from build123d import *

# Parameters (mm, degrees)
BOSS_EXTRUDE1_DEPTH = 15
FILLET1_R           = 5
FILLET2_R           = 5
SKETCH4_W           = 5
SKETCH4_H           = 5
BOSS_EXTRUDE2_DEPTH = 15
SKETCH6_W           = 15
SKETCH6_H           = 35
BOSS_EXTRUDE3_DEPTH = 5
FILLET3_R           = 5
CHAMFER1_SIZE       = 10
BOSS_EXTRUDE4_DEPTH = 5
SKETCH9_R           = 8
CUT_EXTRUDE6_DEPTH  = 5


with BuildPart() as part:
    # Sketch1 → Boss-Extrude1 (new body, symmetric)
    with BuildSketch(Plane.YZ):
        Polygon((45, 0), (45, 5), (25, 5), (25, 50), (0, 50), (0, 45), (20, 45), (20, 0), align=None)
    extrude(amount=BOSS_EXTRUDE1_DEPTH, both=True)

    # Fillet1
    fillet1_edges = [part.edges().sort_by_distance(p)[0] for p in [
        (0, 25, 5),
    ]]
    fillet(fillet1_edges, radius=FILLET1_R)

    # Fillet2
    fillet2_edges = [part.edges().sort_by_distance(p)[0] for p in [
        (0, 20, 0),
        (0, 20, 45),
        (0, 25, 50),
    ]]
    fillet(fillet2_edges, radius=FILLET2_R)

    # Sketch4 → Boss-Extrude2 (add)
    with BuildSketch(Plane(origin=(0, 0, 0), x_dir=(-1, 0, 0), z_dir=(0, 1, 0))):
        with Locations((17.5, 47.5)):
            Rectangle(SKETCH4_W, SKETCH4_H)
    extrude(amount=BOSS_EXTRUDE2_DEPTH)

    # Sketch6 → Boss-Extrude3 (add)
    with BuildSketch(Plane(origin=(-20, 0, 0), x_dir=(0, -1, 0), z_dir=(-1, 0, 0))):
        with Locations((-7.5, 62.5)):
            Rectangle(SKETCH6_W, SKETCH6_H)
    extrude(amount=BOSS_EXTRUDE3_DEPTH)

    # Fillet3
    fillet3_edges = [part.edges().sort_by_distance(p)[0] for p in [
        (-25, 7.5, 45),
        (-20, 7.5, 50),
    ]]
    fillet(fillet3_edges, radius=FILLET3_R)

    # Chamfer1
    chamfer1_edges = [part.edges().sort_by_distance(p)[0] for p in [
        (-22.5, 15, 80),
    ]]
    chamfer(chamfer1_edges, length=CHAMFER1_SIZE)

    # Sketch8 → Boss-Extrude4 (add)
    with BuildSketch(Plane.XY.offset(5)):
        with BuildLine():
            Line((-15, 45), (15, 45))
            ThreePointArc((15, 45), (0, 60), (-15, 45))
        make_face()
    extrude(amount=-BOSS_EXTRUDE4_DEPTH)

    # Sketch9 → Cut-Extrude6 (cut)
    with BuildSketch(Plane.XY.offset(5)):
        with Locations((0, 45)):
            Circle(SKETCH9_R)
    extrude(amount=-CUT_EXTRUDE6_DEPTH, mode=Mode.SUBTRACT)

    # Mirror2: part across plane


with BuildPart() as part_1:
    add(part.part)
    add(part.part.mirror(Plane(origin=(15, 0, 50), x_dir=(0, 0, 1), z_dir=(0, 1, 0))))


solid = part_1.part
Input: part model. Units: mm. Frame: model coordinates. A direction names the side the tool comes from. Give positions to 0.01 mm unless a question says otherwise; leave off trailing zeros. Write each loop counter-clockwise with the first axis right and the second up, starting at its lowest first coordinate (ties: lowest second). Pieces come first, ordered by that corner, then holes. Notation, with made-up numbers: (-40, 18) -> (1, 18) arc R24 ccw to (1, 43) -> close; hole circle Ø7 at (-27, 71). An arc over 180 degrees is marked (long way). Use one line per item in the form item = value. Start each with the question number.
1) Section query A-A on x = 0. Return the cut outline in (y, z).
2) Set-up query: faces 1 (the cylindrical face through (0, 19, 43)), 2 (the flat face through (-20, 0, 65)), 3 (the flat face through (-15, -24, 20)), 4 (the flat face through (-15, 24, 20)), 5 (the flat face through (0, -25, 27)). Return all of +Z, -Z, +X, -X, +Y, -Y with unobstructed straight access to the full face (end or side cutting, diameter ignored); none if empty.
3) Section query B-B on y = -43.5. Return the cut outline in (x, z).
4) Ray query, probe 1 along Y at (x, z) = (0, 3.25); probe 2 along Y at (x, z) = (0, 1.35); probe 3 along Y at (x, z) = (1, 20.5). Return the intervals inside material, ascending. Write a range as from..to.
5) Section query D-D on z = 47.5. Return the cut outline in (x, y), then the cut area to 3 significant figures.
6) Section query C-C on y = 9. Return the cut outline in (x, z).
7) Pin query (flat end, axial travel): pin 1 (5 mm diameter, centred on x = -21, z = 55.5, fed in from -Y); pin 2 (5 mm diameter, centred on x = -22.5, z = 63.5, fed in from +Y); pin 3 (3 mm diameter, centred on x = -5.5, y = 15, fed in from +Z). Return the tip coordinate at first contact, or that it passes through.
8) Draft query along X for faces 6 (the cylindrical face through (0, -19, 43)), 7 (the cylindrical face through (0, 60, 3)), 8 (the cylindrical face through (-1.041, 52.932, 2.535)). Return one class per face: pulls with the +X half, pulls with the -X half, needs draft (parallel to the pull), parting line crosses it, or undercut.
Outcome:
q1.outline = (-60, 0) -> (-53, 0) -> (-53, 5) -> (-60, 5) -> close; (-37, 0) -> (-25, 0) arc R5 ccw to (-20, 5) -> (-20, 40) arc R5 cw to (-15, 45) -> (15, 45) arc R5 cw to (20, 40) -> (20, 5) arc R5 ccw to (25, 0) -> (37, 0) -> (37, 5) -> (30, 5) arc R5 cw to (25, 10) -> (25, 45) arc R5 ccw to (20, 50) -> (-20, 50) arc R5 ccw to (-25, 45) -> (-25, 10) arc R5 cw to (-30, 5) -> (-37, 5) -> close; (53, 0) -> (60, 0) -> (60, 5) -> (53, 5) -> close
q2.face_1 = -Z, +X, -X
q2.face_2 = +Z, +X, +Y, -Y
q2.face_3 = +Z, -Z, -X, -Y
q2.face_4 = +Z, -Z, -X, +Y
q2.face_5 = +Z, +X, -X, -Y
q3.outline = (-15, 0) -> (-7.86, 0) -> (-7.86, 5) -> (-15, 5) -> close; (7.86, 0) -> (15, 0) -> (15, 5) -> (7.86, 5) -> close
q4.probe_1 = -60..-53, -37..-20.32, 20.32..37, 53..60
q4.probe_2 = -60..-53, -37..-21.58, 21.58..37, 53..60
q4.probe_3 = -25..-20, 20..25
q5.outline = (-24.33, -15) -> (-15, -15) -> (-15, -24.33) -> (15, -24.33) -> (15, 24.33) -> (-15, 24.33) -> (-15, 15) -> (-24.33, 15) -> close
q5.area = 1,740 mm^2
q6.outline = (-25, 50) arc R5 ccw to (-20, 45) -> (15, 45) -> (15, 50) -> (-15, 50) arc R5 cw to (-20, 55) -> (-20, 76) -> (-25, 76) -> close
q7.pin_1 = -15
q7.pin_2 = 15
q7.pin_3 = 50
q8.face_6 = needs draft
q8.face_7 = parting line crosses it
q8.face_8 = undercut
